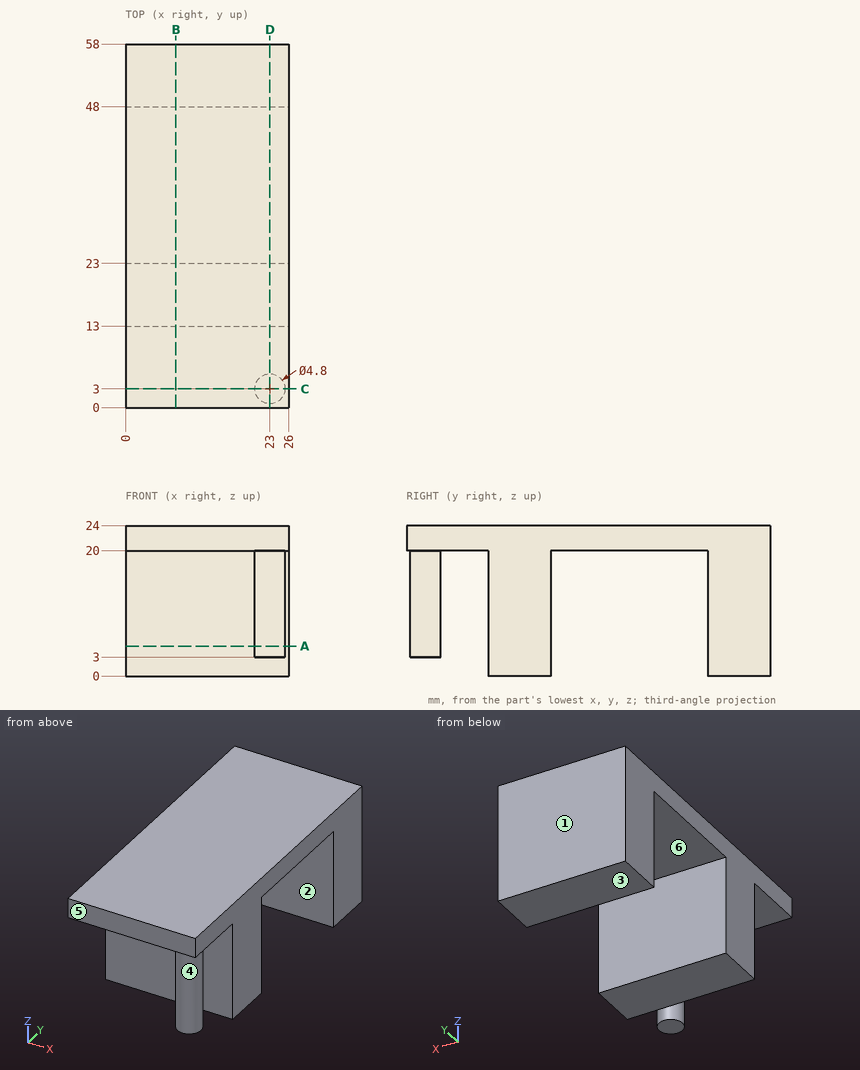
Design review of the part shown in the three views and the two pictorial views. Dimensions are in mm from the part's minimum x, y and z. A direction names the side the tool comes from. Round coordinates to 2 decimals unless told otherwise and drop trailing zeros. Loops run counter-clockwise (first coordinate to the right, second up) from the corner with the lowest first, then second, coordinate; pieces in that order, holes last. Notation, with made-up numbers: (84, 15.25) -> (128, 15.25) arc R25 cw to (128, 48.25) -> close; hole circle Ø11 at (56.25, 21.5). An arc over 180 degrees is marked (long way). Answer as a JSON object with one key per item and string values. Group by question number.
1) We need section A-A on z = 4.75. Write out the cut boundary in (x, y).
2) We need section B-B on x = 8. Write out the cut boundary in (y, z).
3) We need section C-C on y = 3. Write out the cut boundary in (x, z).
4) For the marked faces 4, 5 and 6, list the 3-axis set-ups (+Z, -Z, +X, -X, +Y, -Y) from which the entire face can be reached by the end or side of a thin tool; tool diameter is ignored.
5) We need section D-D on x = 23. Write out the cut boundary in (y, z), then the cut area to 3 significant figures.
6) For line 1 (Y direction, x = 13, z = 5.25); line 2 (Y direction, x = 21.5, z = 18); line 3 (Z direction, x = 17.5, y = 46), list the stretches that pass through material, from the lowest coordinate up. Write a range as [from, to].
7) Mouldability with a two-part tool opening along Y and no side actions: class the marked faces 1, 2 and 3 as released by +Y, released by -Y, zero draft, split by the parting line, or undercut.
8) For pin 1 Ø5 at (x, z) = (19, 5.5) entering from -Y; pin 2 Ø4 at (x, z) = (9, 11.5) entering from -Y; pin 3 Ø1.5 at (x, y) = (20.5, 46.5) entering from -Z, all flat-tipped, find the tip position at first contact; note any pin that passes through.
Result set:
{
 "1": {"outline": "(0, 13) -> (26, 13) -> (26, 23) -> (0, 23) -> close; (0, 48) -> (26, 48) -> (26, 58) -> (0, 58) -> close; circle Ø4.8 at (23, 3)"},
 "2": {"outline": "(0, 20) -> (13, 20) -> (13, 0) -> (23, 0) -> (23, 20) -> (48, 20) -> (48, 0) -> (58, 0) -> (58, 24) -> (0, 24) -> close"},
 "3": {"outline": "(0, 20) -> (20.6, 20) -> (20.6, 3) -> (25.4, 3) -> (25.4, 20) -> (26, 20) -> (26, 24) -> (0, 24) -> close"},
 "4": {"face 4": "-Z", "face 5": "+Z, -Z, +X, -X, -Y", "face 6": "-Z, +X, -X"},
 "5": {"outline": "(0, 20) -> (0.6, 20) -> (0.6, 3) -> (5.4, 3) -> (5.4, 20) -> (13, 20) -> (13, 0) -> (23, 0) -> (23, 20) -> (48, 20) -> (48, 0) -> (58, 0) -> (58, 24) -> (0, 24) -> close", "area": "714 mm²"},
 "6": {"line 1": "[13, 23], [48, 58]", "line 2": "[1.13, 4.87], [13, 23], [48, 58]", "line 3": "[20, 24]"},
 "7": {"face 1": "released by +Y", "face 2": "undercut", "face 3": "zero draft"},
 "8": {"pin 1": "y = 1.13", "pin 2": "y = 13", "pin 3": "z = 20"}
}
